For this review, take the finished solid that the model builds, in its own axes (mm). Face numbers are marked on the shaded views. A direction names the side the tool comes from. Round coordinates to 2 decimals unless told otherwise and drop trailing zeros. Write each loop counter-clockwise with the first axis right and the second up, starting at its lowest first coordinate (ties: lowest second). Pieces come first, ordered by that corner, then holes. Notation, with made-up numbers: (12.25, 88) -> (54.25, 88) arc R31 cw to (54.25, 116) -> close; hole circle Ø6 at (26.25, 34). An arc over 180 degrees is marked (long way). Answer as CSV lines item,"result". Start each with the question number.
Item 1: For pin 1 Ø2.5 at (x, y) = (-34.5, 84.5) entering from -Z, flat-tipped, find the tip position at first contact; note if it passes through.
Item 2: Take a section at C-C on y = 79.5. Give the boundary of the cut face in (x, z) (3 decimals).
Item 3: Take a section at A-A on x = 0. Give the boundary of the cut face in (y, z) (3 decimals).
Item 4: Mouldability with a two-part tool opening along X and no side actions: class the marked faces 1, 2 and 3 as +X half, -X half, draft (parallel to the pull), parting line (faces both ways), or undercut.
Item 5: Wall thickness on probe 1 along Y at (x, z) = (0, 10) (3 decimals); probe 2 along X at (y, z) = (145, 4.75) (3 decimals); probe 3 along X at (y, z) = (146, 9) (3 decimals): over which ranges is each line inside the solid? List them lowest first. Write a range as from..to.
Item 6: Machinability: for the marked faces 4 and 5, which of the approach directions +Z, -Z, +X, -X, +Y, -Y give a long, thin tool a straight path to every point of the face, cutting with its end or side? Answer none if there is none.
Item 7: Take a section at B-B on z = 8.25. Count the separate pieces of the cut face and the enclosed holes in it, then the cut area to 3 significant figures.
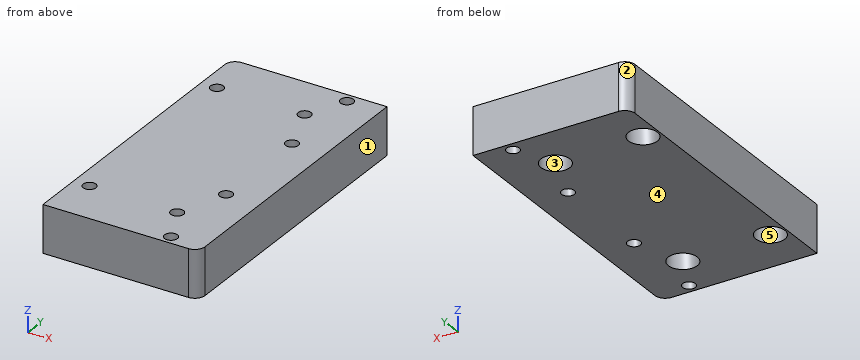
Autodesk Inventor part; units mm, degrees
ref_plane "Work Plane2" through (-72.402, 8.8416, 0) normal (0, 0, 1) x (1, 0, 0)
ref_plane "Work Plane3" through (-84.9315, 9.3639, 0) normal (0, 0, 1) x (1, 0, 0)
ref_plane "YZ Plane" through (0, 0, 0) normal (1, 0, 0) x (0, 1, 0)
ref_plane "Work Plane1" through (-2.3114, 87.1581, 14.5288) normal (0, 0, -1) x (-1, 0, 0)
sketch "Sketch1" plane through (-2.3114, 87.1581, 14.5288) normal (0, 0, -1) x (-1, 0, 0)
  line L0 (0, -9.525) -> (33.4772, -9.525) construction
  line L1 (35.1536, 0) -> (35.1536, -9.525) construction
  line L2 (0, 62.419) -> (33.4772, 62.419) construction
  line L3 (-12.7, -19.685) -> (-12.7, 72.579)
  arc A0 (30.0098, 55.9153) -> (28.8277, 56.5778) centre (30.209, 57.6565) ccw construction
  arc A1 (30.0098, -6.5037) -> (28.8277, -5.8412) centre (30.209, -4.7625) ccw construction
  spline S0 degree 3 poles (-36.5707, 76.7108) (-36.5399, 76.774) (-36.5004, 76.8533) (-36.4067, 77.0384) (-36.3532, 77.143) (-36.2191, 77.4029) (-36.1252, 77.5838) (-35.9667, 77.8845) (-35.9172, 77.9778) (-35.7665, 78.2605) (-35.6659, 78.447) (-35.4766, 78.7937) (-35.4006, 78.9307) (-35.2724, 79.1587) (-35.2158, 79.2566) (-35.126, 79.4049) (-35.0957, 79.4501) (-35.0767, 79.4671) (-35.0747, 79.4643) (-35.0811, 79.4361) (-35.0968, 79.3935) (-35.1824, 79.2047) (-35.234, 79.0957) (-35.3802, 78.7956) (-35.4651, 78.6264) (-35.5969, 78.3654) (-35.6729, 78.2163) (-35.8204, 77.9297) (-35.8907, 77.794) (-36.0446, 77.5001) (-36.107, 77.3829) (-36.1471, 77.3082) knots 0.000001 0.000001 0.000001 0.000001 0.04651 0.04651 0.092381 0.092381 0.150569 0.150569 0.176245 0.176245 0.228297 0.228297 0.280311 0.280311 0.337729 0.337729 0.399083 0.399083 0.42945 0.42945 0.476927 0.476927 0.513851 0.513851 0.562369 0.562369 0.621068 0.621068 0.675896 0.675896 0.74783 0.74783 0.74783 0.74783 construction
  spline S1 degree 3 poles (-36.5707, 14.2918) (-36.5399, 14.355) (-36.5004, 14.4343) (-36.4067, 14.6194) (-36.3532, 14.724) (-36.2191, 14.9839) (-36.1252, 15.1648) (-35.9667, 15.4655) (-35.9172, 15.5588) (-35.7665, 15.8415) (-35.6659, 16.028) (-35.4766, 16.3747) (-35.4006, 16.5117) (-35.2724, 16.7397) (-35.2158, 16.8376) (-35.126, 16.9859) (-35.0957, 17.0311) (-35.0767, 17.0481) (-35.0747, 17.0453) (-35.0811, 17.0171) (-35.0968, 16.9745) (-35.1824, 16.7857) (-35.234, 16.6767) (-35.3802, 16.3766) (-35.4651, 16.2074) (-35.5969, 15.9464) (-35.6729, 15.7973) (-35.8204, 15.5107) (-35.8907, 15.375) (-36.0446, 15.0811) (-36.107, 14.9639) (-36.1471, 14.8892) knots 0.000001 0.000001 0.000001 0.000001 0.04651 0.04651 0.092381 0.092381 0.150569 0.150569 0.176245 0.176245 0.228297 0.228297 0.280311 0.280311 0.337729 0.337729 0.399083 0.399083 0.42945 0.42945 0.476927 0.476927 0.513851 0.513851 0.562369 0.562369 0.621068 0.621068 0.675896 0.675896 0.74783 0.74783 0.74783 0.74783 construction
  circle A2 centre (30.209, -4.7625) radius 1.9685
  circle A3 centre (30.209, 57.6565) radius 1.9685
  arc A4 (3.0691, -6.5037) -> (1.8869, -5.8412) centre (3.2682, -4.7625) ccw construction
  arc A5 (3.0691, 55.9153) -> (1.8869, 56.5778) centre (3.2682, 57.6565) ccw construction
  circle A6 centre (3.2682, 57.6565) radius 1.9685
  circle A7 centre (3.2682, -4.7625) radius 1.9685
  line L4 (35.1536, -19.685) -> (-12.7, -19.685)
  line L5 (35.1536, 72.579) -> (-12.7, 72.579)
  line L6 (35.1536, -19.685) -> (35.1536, 72.579)
  point P0 (-2.3114, -87.1581)
  point P1 (-12.7, 62.419)
  dimension "d0" = 3.937
  dimension "d1" = 3.937
  dimension "d4" = 3.937
  dimension "d5" = 3.937
ref_plane "Work Plane2" through (-72.402, 8.8416, 0) normal (0, 0, 1) x (1, 0, 0)
ref_plane "Work Plane3" through (-84.9315, 9.3639, 0) normal (0, 0, 1) x (1, 0, 0)
extrude "Extrusion2" add sketch "Sketch1" along normal up to surface (14.5288 mm away)
sketch "Sketch2" plane through (10.3886, 77.6331, 0) normal (0, 0, -1) x (-1, 0, 0)
  circle A0 centre (42.909, 4.7625) radius 1.9685
  circle A1 centre (42.909, 4.7625) radius 1.9685
  circle A2 centre (42.909, 67.1815) radius 1.9685
  circle A3 centre (42.909, 67.1815) radius 1.9685
  circle A4 centre (15.9682, 4.7625) radius 1.9685
  circle A5 centre (15.9682, 4.7625) radius 1.9685
  circle A6 centre (15.9682, 67.1815) radius 1.9685
  circle A7 centre (15.9682, 67.1815) radius 1.9685
  point P0 (10.3886, -77.6331)
  dimension "d12" = 3.937
  dimension "d13" = 3.937
  dimension "d14" = 3.937
  dimension "d15" = 3.937
hole "Hole1" at (-5.5796, 144.8146, 0) at (-32.5204, 144.8146, 0) at (-32.5204, 82.3956, 0) at (-5.5796, 82.3956, 0) direction (0, 0, 1) diameter 3.937 end through all counterbore diameter 8.89 counterbore depth 5.08
sketch "Sketch3" plane through (-2.3114, 87.1581, 14.5288) normal (0, 0, 1) x (1, 0, 0)
  arc A0 (3.5282, -17.9067) -> (2.2941, -18.3979) centre (2.3114, -16.6454) ccw construction
  arc A1 (3.5282, 9.034) -> (2.2941, 8.5429) centre (2.3114, 10.2954) ccw construction
  arc A2 (3.5282, 41.3373) -> (2.2941, 40.8461) centre (2.3114, 42.5986) ccw construction
  arc A3 (3.5282, 68.278) -> (2.2941, 67.7869) centre (2.3114, 69.5394) ccw construction
  circle A4 centre (2.3114, -16.6454) radius 1.9685
  circle A5 centre (2.3114, 10.2954) radius 1.9685
  circle A6 centre (2.3114, 42.5986) radius 1.9685
  circle A7 centre (2.3114, 69.5394) radius 1.9685
  point P0 (2.3114, -87.1581)
  dimension "d37" = 3.937
  dimension "d38" = 3.937
  dimension "d39" = 3.937
  dimension "d40" = 3.937
hole "Hole2" at (0, 70.5127, 14.5288) at (0, 97.4535, 14.5288) at (0, 129.7567, 14.5288) at (0, 156.6975, 14.5288) direction (0, 0, -1) diameter 3.937 end through all
fillet "Fillet1" radius 3.175 2 edges at (10.3886, 67.4731, 7.2644) (-37.465, 159.7371, 7.2644)
properties part number "RightAngleMotorMountExtensionArm"
Output values:
1,pin 1,"stops at z = 5.08"
2,outline,"(-37.465, 0) -> (-35.893, 0) -> (-35.893, 5.08) -> (-29.148, 5.08) -> (-29.148, 0) -> (-8.952, 0) -> (-8.952, 5.08) -> (-2.207, 5.08) -> (-2.207, 0) -> (10.389, 0) -> (10.389, 14.529) -> (-37.465, 14.529) -> close"
3,outline,"(67.473, 0) -> (68.544, 0) -> (68.544, 14.529) -> (67.473, 14.529) -> close; (72.481, 0) -> (95.485, 0) -> (95.485, 14.529) -> (72.481, 14.529) -> close; (99.422, 0) -> (127.788, 0) -> (127.788, 14.529) -> (99.422, 14.529) -> close; (131.725, 0) -> (154.729, 0) -> (154.729, 14.529) -> (131.725, 14.529) -> close; (158.666, 0) -> (159.737, 0) -> (159.737, 14.529) -> (158.666, 14.529) -> close"
4,face 1,"+X half"
4,face 2,"-X half"
4,face 3,"undercut"
5,probe 1,"y = 67.473..68.544, 72.481..95.485, 99.422..127.788, 131.725..154.729, 158.666..159.737"
5,probe 2,"x = -37.465..-36.962, -28.079..-10.021, -1.138..10.389"
5,probe 3,"x = -37.465..-34.092, -30.949..-7.151, -4.008..10.389"
6,face 4,"-Z, +X, -X, +Y, -Y"
6,face 5,"-Z"
7,separate pieces,"1"
7,enclosed holes,"8"
7,area,"4,310 mm^2"
